Build history of the part. All positions in model axes, mm. Face numbers are marked on the shaded views. A direction names the side the tool comes from. Give positions to 0.01 mm unless a question says otherwise; leave off trailing zeros. Write each loop counter-clockwise with the first axis right and the second up, starting at its lowest first coordinate (ties: lowest second). Pieces come first, ordered by that corner, then holes. Notation, with made-up numbers: (41.5, 56) -> (55.5, 56) arc R19 ccw to (55.5, 79) -> close; hole circle Ø10 at (34, -18). An arc over 180 degrees is marked (long way). Put each result on its own line as item: value.
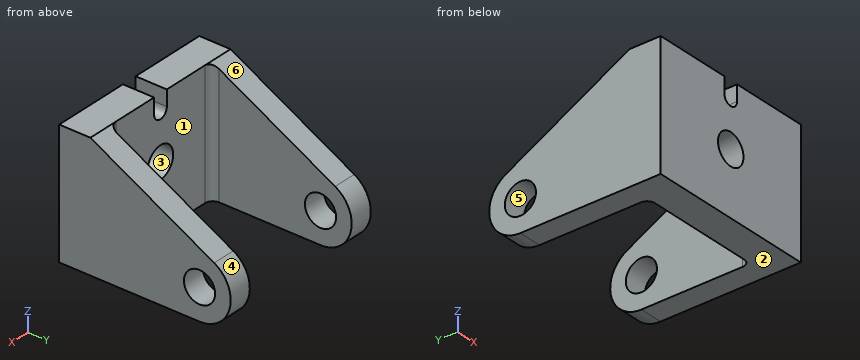
from build123d import *

# Parameters (mm, degrees)
SKETCH1_W           = 69.85
SKETCH1_H           = 50.8
BOSS_EXTRUDE1_DEPTH = 12.7
BOSS_EXTRUDE2_START = 34.925
SKETCH2_R           = 6.35
BOSS_EXTRUDE2_DEPTH = 9.525
BOSS_EXTRUDE3_START = -25.4
SKETCH2_2_R         = 6.35
BOSS_EXTRUDE3_DEPTH = 9.525
SKETCH3_R           = 6.35
CUT_EXTRUDE1_DEPTH  = 72.631264997
FILLET2_R           = 3.175


with BuildPart() as part:
    # Sketch1 → Boss-Extrude1 (new body)
    with BuildSketch(Plane(origin=(0, 0, 0), x_dir=(1, 0, 0), z_dir=(0, 1, 0))):
        Rectangle(SKETCH1_W, SKETCH1_H)
    extrude(amount=BOSS_EXTRUDE1_DEPTH)

    # Sketch2 → Boss-Extrude2 (add)
    with BuildSketch(Plane(origin=(0, 0, 0), x_dir=(0, 0, -1), z_dir=(1, 0, 0)).offset(BOSS_EXTRUDE2_START)):
        with BuildLine():
            Line((-25.4, 12.7), (1.494117647, 63.126470588))
            ThreePointArc((1.494117647, 63.126470588), (15.780202438, 69.470809752), (25.4, 57.15))
            Line((25.4, 57.15), (25.4, 12.7))
            Line((25.4, 12.7), (-25.4, 12.7))
        make_face()
        with Locations((12.7, 57.15)):
            Circle(SKETCH2_R, mode=Mode.SUBTRACT)
    extrude(amount=-BOSS_EXTRUDE2_DEPTH)

    # Sketch2<2> → Boss-Extrude3 (add)
    with BuildSketch(Plane(origin=(0, 0, 0), x_dir=(0, 0, -1), z_dir=(1, 0, 0)).offset(BOSS_EXTRUDE3_START)):
        with BuildLine():
            Line((-25.4, 12.7), (1.494117647, 63.126470588))
            ThreePointArc((1.494117647, 63.126470588), (15.780202438, 69.470809752), (25.4, 57.15))
            Line((25.4, 57.15), (25.4, 12.7))
            Line((25.4, 12.7), (-25.4, 12.7))
        make_face()
        with Locations((12.7, 57.15)):
            Circle(SKETCH2_2_R, mode=Mode.SUBTRACT)
    extrude(amount=-BOSS_EXTRUDE3_DEPTH)

    # Sketch3 → Cut-Extrude1 (cut, through all)
    with BuildSketch(Plane(origin=(0, 12.7, 0), x_dir=(1, 0, 0), z_dir=(0, 1, 0))):
        with Locations(Location((0, 0, 0), (0, 0, 270))):
            Circle(SKETCH3_R)
        with BuildLine():
            Line((3.175, -19.05), (3.175, -25.4))
            Line((3.175, -25.4), (-3.175, -25.4))
            Line((-3.175, -25.4), (-3.175, -19.05))
            ThreePointArc((-3.175, -19.05), (0, -15.875), (3.175, -19.05))
        make_face()
    extrude(amount=-CUT_EXTRUDE1_DEPTH, mode=Mode.SUBTRACT)

    # Fillet2
    fillet2_edges = [part.edges().sort_by_distance(p)[0] for p in [
        (25.4, 12.7, 0),
        (-25.4, 12.7, 0),
    ]]
    fillet(fillet2_edges, radius=FILLET2_R)


solid = part.part
1) Tool access for the marked faces 1 and 2: list every direction of +Z, -Z, +X, -X, +Y, -Y with a clear straight run to the whole face (end or side of a thin tool).
Filled sheet:
face 1: +Z, -Z, +Y
face 2: -Z, +X, -X, +Y, -Y
2) Slice it at A-A (y = 41.5). Write the cut outline in (x, z) (3 decimals), plus the area to 3 significant figures.
Filled sheet:
outline: (-34.925, -25.4) -> (-25.4, -25.4) -> (-25.4, 10.04) -> (-34.925, 10.04) -> close; (25.4, -25.4) -> (34.925, -25.4) -> (34.925, 10.04) -> (25.4, 10.04) -> close
area: 675 mm2
3) Slice it at B-B (z = -12.7). Write the cut outline in (x, y) (3 decimals).
Filled sheet:
outline: (-34.925, 0) -> (34.925, 0) -> (34.925, 50.8) -> (25.4, 50.8) -> (25.4, 15.875) arc R3.175 cw to (22.225, 12.7) -> (-22.225, 12.7) arc R3.175 cw to (-25.4, 15.875) -> (-25.4, 50.8) -> (-34.925, 50.8) -> close; (-34.925, 63.5) -> (-25.4, 63.5) -> (-25.4, 69.85) -> (-34.925, 69.85) -> close; (25.4, 63.5) -> (34.925, 63.5) -> (34.925, 69.85) -> (25.4, 69.85) -> close
4) Pull direction Z, two halves, no side cores. Call the marked faces 3, 4, 5 and 6: released by +Z, released by -Z, zero draft, split by the parting line, or undercut.
Filled sheet:
face 3: undercut
face 4: split by the parting line
face 5: undercut
face 6: released by +Z
5) Slice it at D-D (x = 28.5). Write the cut outline in (y, z), plus the area to 3 significant figures.
Filled sheet:
outline: (0, -25.4) -> (57.15, -25.4) arc R12.7 ccw to (63.13, -1.49) -> (12.7, 25.4) -> (0, 25.4) -> close; hole circle Ø12.7 at (57.15, -12.7)
area: 2,510 mm2
6) Wall check: L1, parallel to X at y = 41.5, z = -20.5 (3 decimals); L2, parallel to X at y = 8.5, z = 0 (3 decimals); L3, parallel to Y at x = -5, z = -11. Give the ranges that are in metal, low to high.
Filled sheet:
L1: -34.925 to -25.4, 25.4 to 34.925
L2: -34.925 to -6.35, 6.35 to 34.925
L3: 0 to 12.7
7) Pin check, flat tip, straight feed: pin 1 (1 mm diameter, centred on x = 15, z = 5.5, fed in from +Y). Stop position of the tip, or through.
Filled sheet:
pin 1: y = 12.7
